Geometry check sheet. Reference: the model listing, model coordinates, mm. Give positions to 0.01 mm unless a question says otherwise; leave off trailing zeros. Loops run counter-clockwise (first coordinate to the right, second up) from the corner with the lowest first, then second, coordinate; pieces in that order, holes last. Notation, with made-up numbers: (68, 65.25) -> (116, 65.25) arc R20 cw to (116, 79.25) -> close; hole circle Ø2 at (31, 69). An arc over 180 degrees is marked (long way). Answer in a Markdown table with one row per item. Add a question column.
Autodesk Inventor part; units mm, degrees
ref_plane "YZ Plane" through (0, 0, 0) normal (1, 0, 0) x (0, 1, 0)
ref_plane "XZ Plane" through (0, 0, 0) normal (0, 1, 0) x (-1, 0, 0)
ref_plane "XY Plane" through (0, 0, 0) normal (0, 0, 1) x (1, 0, 0)
sketch "Sketch1" plane through (0, 0, 0) normal (0, 0, 1) x (1, 0, 0)
  circle A0 centre (7.5, -10) radius 2
  circle A1 centre (7.5, -60) radius 2
  line L0 (0, 0) -> (0, -69.9999)
  line L1 (0, -69.9999) -> (15, -69.9999)
  line L2 (15, 0) -> (15, -69.9999)
  line L3 (0, 0) -> (15, 0)
  line L4 (15, 0) -> (-85, 0)
  line L5 (-85, 0) -> (-85, -70)
  line L6 (-85, -70) -> (15, -70)
  line L7 (15, -70) -> (15, 0)
  circle A2 centre (-77.5, -10) radius 2
  circle A3 centre (-77.5, -60) radius 2
  line L8 (-85, 0) -> (-85, -69.9999)
  line L9 (-85, -69.9999) -> (-70, -69.9999)
  line L10 (-70, 0) -> (-70, -69.9999)
  line L11 (-85, 0) -> (-70, 0)
  dimension "d0" = 100
  dimension "d1" = 70
extrude "Extrusion1" add sketch "Sketch1" along normal blind 2
properties part number "Copper_Plate" material "Copper"
1. Material ranges on L1, parallel to Y at x = 7.5, z = 0.7; L2, parallel to X at y = -61.5, z = 1.55, recorded low to high. Write a range as from..to.
2. Sectioned sample at B-B (y = -10). Enter the section's corners in (x, z), plus the area to 3 significant figures.
3. Release check for a two-part mould opening along Y. For faces 1 (the face through (-36, 0, 1)), 2 (the face through (15, -35, 1)), 3 (the face through (-76.425, -61.686, 0.986)) record: released by +Y, released by -Y, zero draft, split by the parting line, or undercut.
4. Sectioned sample at A-A (x = -77.5). Enter the section's corners in (y, z), plus the area to 3 significant figures.
Response:
| question | item | result |
|---|---|---|
| 1 | L1 | y = -70..-62, -58..-12, -8..0 |
| 1 | L2 | x = -85..-78.82, -76.18..6.18, 8.82..15 |
| 2 | outline | (-85, 0) -> (-79.5, 0) -> (-79.5, 2) -> (-85, 2) -> close; (-75.5, 0) -> (5.5, 0) -> (5.5, 2) -> (-75.5, 2) -> close; (9.5, 0) -> (15, 0) -> (15, 2) -> (9.5, 2) -> close |
| 2 | area | 184 mm2 |
| 3 | face 1 | released by +Y |
| 3 | face 2 | zero draft |
| 3 | face 3 | undercut |
| 4 | outline | (-70, 0) -> (-62, 0) -> (-62, 2) -> (-70, 2) -> close; (-58, 0) -> (-12, 0) -> (-12, 2) -> (-58, 2) -> close; (-8, 0) -> (0, 0) -> (0, 2) -> (-8, 2) -> close |
| 4 | area | 124 mm2 |
